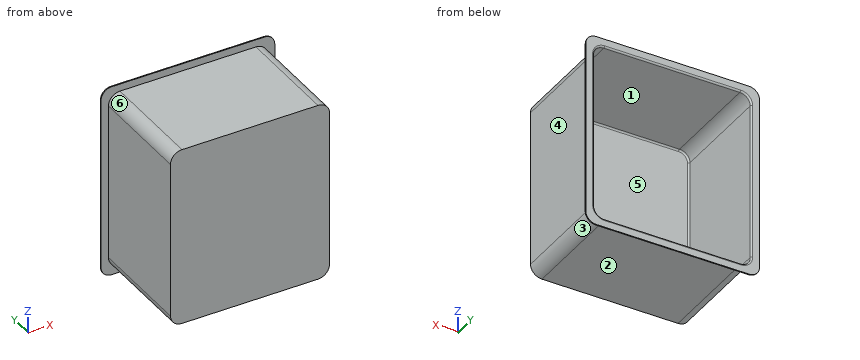
from build123d import *

# Parameters (mm, degrees)
BOSS_EXTRUDE1_DEPTH = 2
CUT_EXTRUDE1_REACH  = 251.311
BOSS_EXTRUDE2_DEPTH = 200
BOSS_EXTRUDE3_DEPTH = 2
FILLET1_R           = 3


with BuildPart() as part:
    # Sketch1 → Boss-Extrude1 (new body)
    with BuildSketch(Plane(origin=(0, 0, 0), x_dir=(1, 0, 0), z_dir=(0, 1, 0))):
        with BuildLine():
            Line((-146, 186), (146, 186))
            ThreePointArc((146, 186), (160.142135624, 180.142135624), (166, 166))
            Line((166, 166), (166, -166))
            ThreePointArc((166, -166), (160.142135624, -180.142135624), (146, -186))
            Line((146, -186), (-146, -186))
            ThreePointArc((-146, -186), (-160.142135624, -180.142135624), (-166, -166))
            Line((-166, -166), (-166, 166))
            ThreePointArc((-166, 166), (-160.142135624, 180.142135624), (-146, 186))
        make_face()
    extrude(amount=BOSS_EXTRUDE1_DEPTH)

    # Sketch2 → Cut-Extrude1 (cut, up to next)
    with BuildSketch(Plane(origin=(0, 2, 0), x_dir=(1, 0, 0), z_dir=(0, 1, 0)), mode=Mode.PRIVATE) as cut_extrude1_sk1:
        with BuildLine():
            Line((-130, 170), (130, 170))
            ThreePointArc((130, 170), (144.142135624, 164.142135624), (150, 150))
            Line((150, 150), (150, -150))
            ThreePointArc((150, -150), (144.142135624, -164.142135624), (130, -170))
            Line((130, -170), (-130, -170))
            ThreePointArc((-130, -170), (-144.142135624, -164.142135624), (-150, -150))
            Line((-150, -150), (-150, 150))
            ThreePointArc((-150, 150), (-144.142135624, 164.142135624), (-130, 170))
        make_face()
    cut_extrude1_tool1 = extrude(cut_extrude1_sk1.sketch, amount=-CUT_EXTRUDE1_REACH, mode=Mode.PRIVATE) & part.part
    add(cut_extrude1_tool1.solids().sort_by_distance((0, 2, 0))[0], mode=Mode.SUBTRACT)

    # Sketch3 → Boss-Extrude2 (add)
    with BuildSketch(Plane.XZ):
        with BuildLine():
            Line((-152, 150), (-152, -150))
            ThreePointArc((-152, -150), (-145.556349186, -165.556349186), (-130, -172))
            Line((-130, -172), (130, -172))
            ThreePointArc((130, -172), (145.556349186, -165.556349186), (152, -150))
            Line((152, -150), (152, 150))
            ThreePointArc((152, 150), (145.556349186, 165.556349186), (130, 172))
            Line((130, 172), (-130, 172))
            ThreePointArc((-130, 172), (-145.556349186, 165.556349186), (-152, 150))
        make_face()
        with BuildLine():
            Line((-130, 170), (130, 170))
            ThreePointArc((130, 170), (144.142135624, 164.142135624), (150, 150))
            Line((150, 150), (150, -150))
            ThreePointArc((150, -150), (144.142135624, -164.142135624), (130, -170))
            Line((130, -170), (-130, -170))
            ThreePointArc((-130, -170), (-144.142135624, -164.142135624), (-150, -150))
            Line((-150, -150), (-150, 150))
            ThreePointArc((-150, 150), (-144.142135624, 164.142135624), (-130, 170))
        make_face(mode=Mode.SUBTRACT)
    extrude(amount=BOSS_EXTRUDE2_DEPTH)

    # Sketch4 → Boss-Extrude3 (add)
    with BuildSketch(Plane.XZ.offset(200)):
        with BuildLine():
            Line((-130, 172), (130, 172))
            ThreePointArc((130, 172), (145.556349186, 165.556349186), (152, 150))
            Line((152, 150), (152, -150))
            ThreePointArc((152, -150), (145.556349186, -165.556349186), (130, -172))
            Line((130, -172), (-130, -172))
            ThreePointArc((-130, -172), (-145.556349186, -165.556349186), (-152, -150))
            Line((-152, -150), (-152, 150))
            ThreePointArc((-152, 150), (-145.556349186, 165.556349186), (-130, 172))
        make_face()
    extrude(amount=BOSS_EXTRUDE3_DEPTH)

    # Fillet1
    fillet1_edges = [part.edges().sort_by_distance(p)[0] for p in [
        (-144.142135624, 2, 164.142135624),
        (0, 2, 170),
        (144.142135624, 2, 164.142135624),
        (150, 2, 0),
        (144.142135624, 2, -164.142135624),
        (0, 2, -170),
        (-144.142135624, 2, -164.142135624),
        (-150, 2, 0),
        (-144.142135624, -200, -164.142135624),
        (0, -200, -170),
        (144.142135624, -200, -164.142135624),
        (150, -200, 0),
        (144.142135624, -200, 164.142135624),
        (0, -200, 170),
        (-144.142135624, -200, 164.142135624),
        (-150, -200, 0),
    ]]
    fillet(fillet1_edges, radius=FILLET1_R)


solid = part.part
Geometry check sheet. Reference: the model listing, model coordinates, mm. Face numbers are marked on the shaded views. A direction names the side the tool comes from. Round coordinates to 2 decimals unless told otherwise and drop trailing zeros. Loops run counter-clockwise (first coordinate to the right, second up) from the corner with the lowest first, then second, coordinate; pieces in that order, holes last.
Item 1: Cross-section at C-C on z = -140. Record the boundary of the cut face in (x, y).
Item 2: Access from +Z, -Z, +X, -X, +Y, -Y to the whole of each face (thin tool, end or side, straight path). Record for the marked faces 4, 5 and 6.
Item 3: Thickness scan on line 1 (Z direction, x = 55, y = -12.5); line 2 (X direction, y = -73.5, z = -92.5); line 3 (Y direction, x = 102.5, z = 57). Record the ranges inside material, lowest first.
Item 4: Cross-section at A-A on y = -77.5. Record the boundary of the cut face in (x, z).
Item 5: Cross-section at B-B on x = 57.5. Record the boundary of the cut face in (y, z).
Item 6: Gauge pin test, flat ends, axial feed: pin 1 (8 mm diameter, centred on x = -107.5, y = -68, fed in from -Z); pin 2 (1.5 mm diameter, centred on x = 57.5, y = -131, fed in from +Z); pin 3 (2 mm diameter, centred on y = -84.5, z = 64, fed in from +X). Record the tip position at first contact, or that the pin passes through.
Item 7: Mould release check, pull along X, two halves, no side actions. Record for the marked faces 1, 2 and 3: pulls with the +X half, pulls with the -X half, needs draft (parallel to the pull), parting line crosses it, or undercut.
Answer sheet:
1. outline: (-166, 0) - (-152, 0) - (-152, -202) - (152, -202) - (152, 0) - (166, 0) - (166, 2) - (153, 2) arc R3 ccw to (150, -1) - (150, -197) arc R3 cw to (147, -200) - (-147, -200) arc R3 cw to (-150, -197) - (-150, -1) arc R3 ccw to (-153, 2) - (-166, 2) - close
2. face 4: +Z, -Z, +X, -Y
2. face 5: +Y
2. face 6: +Z, -X, -Y
3. line 1: z = -172 to -170, 170 to 172
3. line 2: x = -152 to -150, 150 to 152
3. line 3: y = -202 to -200
4. outline: (-152, -150) arc R22 ccw to (-130, -172) - (130, -172) arc R22 ccw to (152, -150) - (152, 150) arc R22 ccw to (130, 172) - (-130, 172) arc R22 ccw to (-152, 150) - close; hole (-150, -150) arc R20 ccw to (-130, -170) - (130, -170) arc R20 ccw to (150, -150) - (150, 150) arc R20 ccw to (130, 170) - (-130, 170) arc R20 ccw to (-150, 150) - close
5. outline: (-202, -172) - (0, -172) - (0, -186) - (2, -186) - (2, -173) arc R3 ccw to (-1, -170) - (-197, -170) arc R3 cw to (-200, -167) - (-200, 167) arc R3 cw to (-197, 170) - (-1, 170) arc R3 ccw to (2, 173) - (2, 186) - (0, 186) - (0, 172) - (-202, 172) - close
6. pin 1: stops at z = -172
6. pin 2: stops at z = 172
6. pin 3: stops at x = 152
7. face 1: undercut
7. face 2: needs draft
7. face 3: pulls with the +X half
